Geometry check sheet. Reference: the model listing, model coordinates, mm. Face numbers are marked on the shaded views. A direction names the side the tool comes from. Coordinates: 2 decimals unless noted, no trailing zeros. Write each loop counter-clockwise with the first axis right and the second up, starting at its lowest first coordinate (ties: lowest second). Pieces come first, ordered by that corner, then holes. Notation, with made-up numbers: (-19.75, 17.5) -> (-10.75, 17.5) arc R22 cw to (-10.75, 40.5) -> close; hole circle Ø10 at (31, 27.25). An arc over 180 degrees is marked (long way). Answer in a Markdown table with one row per item. Add a question column.
1. Cross-section at A-A on z = -22.85. Record the cut outline in (x, y).
2. Cross-section at B-B on x = -35. Record the cut outline in (y, z).
3. Cross-section at C-C on y = 38. Record the cut outline in (x, z).
4. Depth check by flat-ended pin: P1, Ø1, axis at x = -68, y = 1, coming from the +Z side; P2, Ø18.5, axis at y = 20.5, z = 21.5, coming from the -X side; P3, Ø7.5, axis at x = -45, y = 24.5, coming from the +Z side. Enter the tip coordinate at first touch or a pass-through.
5. Scan lines: L1, parallel to Z at x = -50, y = 10; L2, parallel to X at y = 11.5, z = -38.5; L3, parallel to Z at x = 39, y = 13.5. Record each from-to range of solid material in increasing order. Write a range as from..to.
6. Mould release check, pull along X, two halves, no side actions. Record for the marked faces 1, 2, 3 and 4: pulls with the +X half, pulls with the -X half, needs draft (parallel to the pull), parting line crosses it, or undercut.
7. Cross-section at D-D on x = 36.5. Record the cut outline in (y, z), and give its area (3 significant figures).
8. Set-up check for the marked faces 5, 6 and 7: record each of +Z, -Z, +X, -X, +Y, -Y from which the full face is reachable in a straight line by a thin tool's end or side.
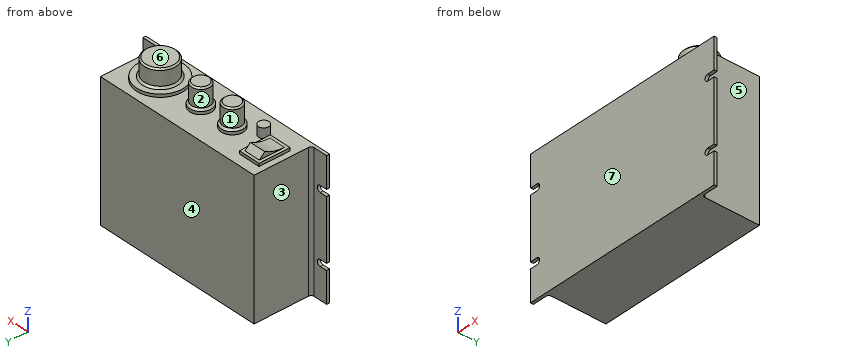
Autodesk Inventor part; units mm, degrees
ref_plane "Work Plane1" through (-52.5, 13, 46) normal (-1, 0, 0) x (0, 0, 1)
ref_plane "Work Plane2" through (-41.5, 13, 46) normal (1, 0, 0) x (0, 0, -1)
ref_plane "YZ Plane" through (0, 0, 0) normal (1, 0, 0) x (0, 1, 0)
sketch "Sketch1" plane through (0, 0, 0) normal (0, 1, 0) x (-1, 0, 0)
  line L0 (70, -46) -> (-70, -46)
  line L1 (-70, -46) -> (-70, 46)
  line L2 (-70, 46) -> (70, 46)
  line L3 (70, 46) -> (70, -46)
  point P0 (0, 0)
  point P1 (0, -46)
  point P2 (-70, 0)
  dimension "d0" = 92
  dimension "d1" = 140
extrude "Extrusion1" add sketch "Sketch1" along normal blind 2
sketch "Sketch2" plane through (0, 2, 0) normal (0, 1, 0) x (1, 0, 0)
  line L0 (70, 46) -> (-70, 46)
  line L1 (-70, 46) -> (-70, -46)
  line L2 (-70, -46) -> (70, -46)
  line L3 (70, -46) -> (70, 46)
  line L4 (70, 46) -> (-70, 46)
  line L5 (-70, -46) -> (70, -46)
  line L6 (-58.5, 46) -> (58.5, 46)
  line L7 (58.5, 46) -> (58.5, -46)
  line L8 (58.5, -46) -> (-58.5, -46)
  line L9 (-58.5, -46) -> (-58.5, 46)
  point P0 (0, 0)
  point P1 (0, 46)
  dimension "d4" = 117
extrude "Extrusion2" add sketch "Sketch2" along normal blind 39 contours L7 L2 L9 L0
fillet "Fillet1" radius 2 2 edges at (58.5, 2, 0) (-58.5, 2, 0)
sketch "Sketch3" plane through (-70, 0, 46) normal (0, 0, 1) x (1, 0, 0)
  line L0 (140, 0) -> (0, 0)
  line L1 (140, 0) -> (140, 2)
  line L2 (130.5, 2) -> (140, 2)
  arc A0 (128.5, 4) -> (130.5, 2) centre (130.5, 4) ccw
  line L3 (128.5, 4) -> (128.5, 41)
  line L4 (11.5, 41) -> (128.5, 41)
  line L5 (11.5, 4) -> (11.5, 41)
  arc A1 (9.5, 2) -> (11.5, 4) centre (9.5, 4) ccw
  line L6 (0, 2) -> (9.5, 2)
  line L7 (0, 0) -> (0, 2)
  circle A2 centre (106.5, 20) radius 16
  circle A3 centre (75, 20.5) radius 7.5
  circle A4 centre (51, 20.5) radius 7.5
  circle A5 centre (35, 13.5) radius 3.5
  line L8 (15.5, 34) -> (30.5, 34)
  line L9 (30.5, 34) -> (30.5, 13)
  line L10 (30.5, 13) -> (15.5, 13)
  line L11 (15.5, 13) -> (15.5, 34)
  point P0 (70, 0)
  dimension "d8" = 32
  dimension "d9" = 15
  dimension "d10" = 15
  dimension "d11" = 7
  dimension "d12" = 15
  dimension "d13" = 21
  dimension "d14" = 4
  dimension "d15" = 7
  dimension "d17" = 10
  dimension "d18" = 20
  dimension "d19" = 13
  dimension "d20" = 32
  dimension "d21" = 13
  dimension "d22" = 56
  dimension "d23" = 4
  dimension "d24" = 6
extrude "Extrusion3" add sketch "Sketch3" along normal blind 2 contours A2 | A3 | A4 | A5 | L8 L9 L10 L11
sketch "Sketch4" plane through (-70, 0, 46) normal (0, 0, 1) x (1, 0, 0)
  circle A0 centre (35, 13.5) radius 3.5
  circle A1 centre (51, 20.5) radius 7.5
  circle A2 centre (75, 20.5) radius 7.5
  circle A3 centre (106.5, 20) radius 16
  circle A4 centre (51, 20.5) radius 6.25
  circle A5 centre (75, 20.5) radius 6.25
  point P0 (70, 0)
  dimension "d28" = 12.5
  dimension "d30" = 12.5
extrude "Extrusion4" add sketch "Sketch4" along normal blind 15.7 contours A4 | A5
sketch "Sketch5" plane through (-70, 0, 46) normal (0, 0, 1) x (1, 0, 0)
  circle A0 centre (106.5, 20) radius 16
  circle A1 centre (106.5, 20) radius 10.85
  point P0 (70, 0)
  dimension "d33" = 21.7
extrude "Extrusion5" add sketch "Sketch5" along normal blind 14 contours A1
sketch "Sketch6" plane through (-70, 0, 46) normal (0, 0, 1) x (1, 0, 0)
  circle A0 centre (35, 13.5) radius 3.5
  circle A1 centre (35, 13.5) radius 3.5
  point P0 (70, 0)
extrude "Extrusion6" add sketch "Sketch6" along normal blind 6.6
chamfer "Chamfer1" distance 1.25 angle 45 3 edges at (25.65, 20, 48) (-1.25, 20.5, 48) (-25.25, 20.5, 48)
chamfer "Chamfer2" distance 1 angle 45 3 edges at (-25.25, 20.5, 61.7) (-1.25, 20.5, 61.7) (25.65, 20, 60)
ref_plane "Work Plane1" through (-52.5, 13, 46) normal (-1, 0, 0) x (0, 0, 1)
ref_plane "Work Plane2" through (-41.5, 13, 46) normal (1, 0, 0) x (0, 0, -1)
sketch "Sketch7" plane through (-52.5, 13, 46) normal (-1, 0, 0) x (0, 0, 1)
  line L0 (0, 0) -> (0, 21)
  line L1 (0, 0) -> (2, 0)
  line L2 (2, 21) -> (2, 0)
  line L3 (0, 21) -> (2, 21)
  line L4 (2, -9) -> (2, 23)
  line L5 (2, 19) -> (2, 2)
  line L6 (2, 19) -> (5.6, 15.4)
  arc A0 (5.6, 15.4) -> (2, 2) centre (28.7389, 2) ccw
  point P0 (-46, -13)
  dimension "d46" = 2
  dimension "d47" = 2
  dimension "d48" = 45
  dimension "d49" = 3.6
extrude "Extrusion7" add sketch "Sketch7" against normal up to surface (11 mm away) contours L2 L6 A0
sketch "Sketch8" plane through (0, 2, 0) normal (0, 1, 0) x (1, 0, 0)
  line L0 (-60.5, 46) -> (-60.5, -46)
  line L1 (-60.5, 46) -> (-70, 46)
  line L2 (-70, 46) -> (-70, -46)
  line L3 (-70, -46) -> (-60.5, -46)
  line L4 (60.5, -46) -> (60.5, 46)
  line L5 (60.5, -46) -> (70, -46)
  line L6 (70, -46) -> (70, 46)
  line L7 (70, 46) -> (60.5, 46)
  line L8 (-70, 46) -> (-70, -46)
  line L9 (-70, 22.85) -> (-65.15, 22.85) construction
  line L10 (-70, 20.7) -> (-65.15, 20.7)
  line L11 (-65.15, 25) -> (-70, 25)
  arc A0 (-70, 25) -> (-70, 20.7) centre (-70, 22.85) ccw
  arc A1 (-65.15, 20.7) -> (-65.15, 25) centre (-65.15, 22.85) ccw
  line L12 (-70, -22.85) -> (-65.15, -22.85) construction
  line L13 (-70, -25) -> (-65.15, -25)
  line L14 (-65.15, -20.7) -> (-70, -20.7)
  arc A2 (-70, -20.7) -> (-70, -25) centre (-70, -22.85) ccw
  arc A3 (-65.15, -25) -> (-65.15, -20.7) centre (-65.15, -22.85) ccw
  line L15 (70, -22.85) -> (65.15, -22.85) construction
  line L16 (70, -25) -> (65.15, -25)
  line L17 (65.15, -20.7) -> (70, -20.7)
  arc A4 (70, -25) -> (70, -20.7) centre (70, -22.85) ccw
  arc A5 (65.15, -20.7) -> (65.15, -25) centre (65.15, -22.85) ccw
  line L18 (70, 46) -> (70, -46)
  line L19 (70, 22.85) -> (65.15, 22.85) construction
  line L20 (70, 20.7) -> (65.15, 20.7)
  line L21 (65.15, 25) -> (70, 25)
  arc A6 (70, 20.7) -> (70, 25) centre (70, 22.85) ccw
  arc A7 (65.15, 25) -> (65.15, 20.7) centre (65.15, 22.85) ccw
  line L22 (70, -46) -> (70, 46)
  point P0 (0, 0)
  point P1 (-67.575, 22.85)
  point P2 (-67.575, -22.85)
  point P3 (67.575, -22.85)
  point P4 (67.575, 22.85)
  dimension "d52" = 4.3
  dimension "d54" = 4.3
  dimension "d55" = 4.3
  dimension "d56" = 7
  dimension "d58" = 7
  dimension "d59" = 7
  dimension "d66" = 4.3
  dimension "d67" = 7
  dimension "d68" = 23.15
  dimension "d69" = 23.15
  dimension "d70" = 23.15
  dimension "d71" = 23.15
extrude "Extrusion8" cut sketch "Sketch8" against normal through all contours L11 A1 L10 L2 | L2 A0 | A2 L2 | L2 L14 A3 L13 | L16 A5 L17 L6 | L6 A4 | A6 L6 | L6 L20 A7 L21
equation "\"d10\" = d9"
equation "\"d21\" = d19"
equation "\"d28\" = d27"
equation "\"d30\" = d28"
equation "\"d54\" = d52"
equation "\"d55\" = d52"
equation "\"d58\" = d56"
equation "\"d59\" = d56"
equation "\"d66\" = d52"
equation "\"d67\" = d56"
equation "\"d69\" = d68"
equation "\"d70\" = d68"
equation "\"d71\" = d68"
properties part number "AmpLP2020A" material "Aluminum 6061"
Results found:
| question | item | result |
|---|---|---|
| 1 | outline | (-63, 0) -> (63, 0) -> (63, 2) -> (60.5, 2) arc R2 cw to (58.5, 4) -> (58.5, 41) -> (-58.5, 41) -> (-58.5, 4) arc R2 cw to (-60.5, 2) -> (-63, 2) -> close |
| 2 | outline | (0, -46) -> (41, -46) -> (41, 46) -> (17, 46) -> (17, 52.6) -> (10, 52.6) -> (10, 46) -> (0, 46) -> close |
| 3 | outline | (-58.5, -46) -> (58.5, -46) -> (58.5, 46) -> (-58.5, 46) -> close |
| 4 | P1 | stops at z = 46 |
| 4 | P2 | stops at x = -58.5 |
| 4 | P3 | stops at z = 51.51 |
| 5 | L1 | z = -46..46 |
| 5 | L2 | x = -58.5..58.5 |
| 5 | L3 | z = -46..60 |
| 6 | face 1 | undercut |
| 6 | face 2 | undercut |
| 6 | face 3 | pulls with the -X half |
| 6 | face 4 | needs draft |
| 7 | outline | (0, -46) -> (41, -46) -> (41, 46) -> (36, 46) -> (36, 48) -> (32.1, 48) -> (30.85, 49.25) -> (30.85, 59) -> (29.85, 60) -> (10.15, 60) -> (9.15, 59) -> (9.15, 49.25) -> (7.9, 48) -> (4, 48) -> (4, 46) -> (0, 46) -> close |
| 7 | area | 4,100 mm^2 |
| 8 | face 5 | +Z, -Z, +X, +Y |
| 8 | face 6 | +Z, +X, +Y, -Y |
| 8 | face 7 | +Z, -Z, +X, -X, -Y |
